Geometry: final body of the model. Coordinates: model frame, mm. Face numbers are marked on the shaded views. A direction names the side the tool comes from. Coordinates: 2 decimals unless noted, no trailing zeros. Loops run counter-clockwise (first coordinate to the right, second up) from the corner with the lowest first, then second, coordinate; pieces in that order, holes last. Notation, with made-up numbers: (3.25, 18) - (25.25, 18) arc R16 cw to (25.25, 23) - close; hole circle Ø3 at (23, 14.5). An arc over 180 degrees is marked (long way). Put each result on its own line as item: value. Start each with the question number.
1) Reachability of the marked faces 5, 6 and 7 from +Z, -Z, +X, -X, +Y, -Y: full face, straight path, thin tool, end or side. Return the list, or none.
2) Section C-C on y = 11. Output: boundary loops of the cut face in (x, z), and give its area (3 significant figures).
3) Material intervals for line 1 along Z through (x, y) = (-5.5, 9.25); line 2 along X through (y, z) = (18, 1), sorted ascending. Write a range as from..to.
4) Section D-D on z = 0. Output: boundary loops of the cut face in (x, y).
5) Section A-A on z = 14.5. Output: boundary loops of the cut face in (x, y).
6) Section B-B on x = -9.5. Output: boundary loops of the cut face in (y, z), and give its area (3 significant figures).
7) Draft query along Z for the marked faces 1, 2, 3 and 4. Return one class per face: +Z half, -Z half, draft (parallel to the pull), parting line (faces both ways), or undercut.
8) Contact query for flat-ended pins moving along their axis: pin 1 Ø23.5 at (x, z) = (-9, 0) entering from +Y; pin 2 Ø22 at (x, z) = (-0.5, 25.5) entering from +Y; pin 3 Ø3 at (x, y) = (-11.5, 21.5) entering from -Z. Output: stop coordinate, or through.
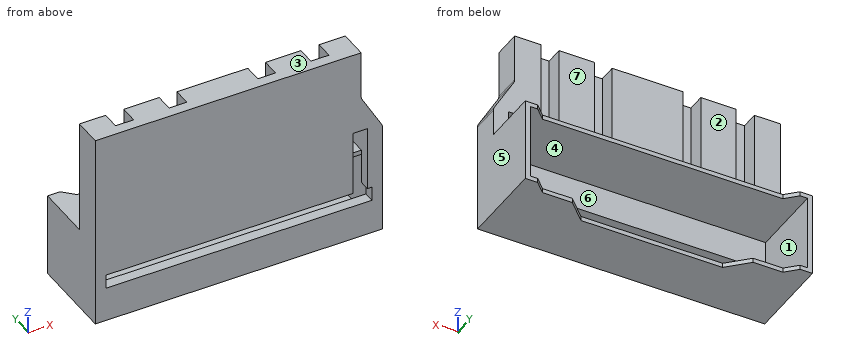
```python
from build123d import *

# Parameters (mm, degrees)
BOSS_EXTRUDE1_DEPTH = 3
SKETCH7_W           = 81
SKETCH7_H           = 23.7
SKETCH7_W_2         = 78.2
SKETCH7_H_2         = 21.2
BOSS_EXTRUDE4_DEPTH = 23.5
CUT_EXTRUDE7_START  = -22.45
CUT_EXTRUDE7_DEPTH  = 22.45
CUT_EXTRUDE8_DEPTH  = 4
CUT_EXTRUDE9_DEPTH  = 4
SKETCH17_W          = 7.4
SKETCH17_H          = 32.3
SKETCH17_W_2        = 10
SKETCH17_W_3        = 20
BOSS_EXTRUDE5_DEPTH = 5
CUT_EXTRUDE10_DEPTH = 1.25
FILLET1_R           = 2


with BuildPart() as part:
    # Sketch1 → Boss-Extrude1 (new body)
    with BuildSketch(Plane(origin=(0, 0, 0), x_dir=(1, 0, 0), z_dir=(0, 1, 0))):
        Polygon((-40.5, -11.85), (-40.5, 11.85), (0, 11.85), (40.5, 11.85), (40.5, -11.85), (40.5, -19.85), (34.5, -30.242304845), (34.5, -44.15), (-40.5, -44.15), align=None)
    extrude(amount=BOSS_EXTRUDE1_DEPTH)

    # Sketch7 → Boss-Extrude4 (add)
    with BuildSketch(Plane(origin=(0, 3, 0), x_dir=(1, 0, 0), z_dir=(0, 1, 0))):
        Rectangle(SKETCH7_W, SKETCH7_H)
        Rectangle(SKETCH7_W_2, SKETCH7_H_2, mode=Mode.SUBTRACT)
    extrude(amount=BOSS_EXTRUDE4_DEPTH)

    # Sketch16 → Cut-Extrude7 (cut)
    with BuildSketch(Plane(origin=(0, 0, -11.85), x_dir=(-1, 0, 0), z_dir=(0, 0, -1)).offset(CUT_EXTRUDE7_START)):
        Polygon((-40.5, 26.5), (40.5, 26.5), (40.5, 24.1), (37, 24.1), (33.9, 21), (25.5, 21), (20, 15.5), (-20, 15.5), (-25.5, 21), (-33.9, 21), (-37, 24.1), (-40.5, 24.1), align=None)
    extrude(amount=CUT_EXTRUDE7_DEPTH, mode=Mode.SUBTRACT)

    # Sketch8 → Cut-Extrude8 (cut)
    with BuildSketch(Plane(origin=(0, 3, 0), x_dir=(1, 0, 0), z_dir=(0, 1, 0))):
        Polygon((33.5, -2), (37.5, -2), (37.5, 2), (-37.5, 2), (-37.5, -2), align=None)
    extrude(amount=-CUT_EXTRUDE8_DEPTH, mode=Mode.SUBTRACT)

    # Sketch14 → Cut-Extrude9 (cut)
    with BuildSketch(Plane(origin=(0, 3, 0), x_dir=(1, 0, 0), z_dir=(0, 1, 0))):
        Polygon((36.25, -11.85), (36.25, -20.35), (32.25, -20.35), (32.25, -11.85), (32.25, 0.15), (36.25, 0.15), align=None)
    extrude(amount=-CUT_EXTRUDE9_DEPTH, mode=Mode.SUBTRACT)

    # Sketch17 → Boss-Extrude5 (add)
    with BuildSketch(Plane(origin=(0, 3, 0), x_dir=(1, 0, 0), z_dir=(0, 1, 0))):
        Polygon((32.25, -20.35), (36.25, -20.35), (36.25, -11.85), (40.5, -11.85), (40.5, -19.85), (34.5, -30.242304845), (34.5, -44.15), (27.1, -44.15), (27.1, -11.85), (32.25, -11.85), align=None)
        with Locations((-36.8, -28)):
            Rectangle(SKETCH17_W, SKETCH17_H)
        with Locations((-23, -28)):
            Rectangle(SKETCH17_W_2, SKETCH17_H)
        with Locations((-3, -28)):
            Rectangle(SKETCH17_W_3, SKETCH17_H)
        with Locations((17, -28)):
            Rectangle(SKETCH17_W_2, SKETCH17_H)
    extrude(amount=BOSS_EXTRUDE5_DEPTH)

    # Sketch18 → Cut-Extrude10 (cut)
    with BuildSketch(Plane(origin=(0, 0, 10.6), x_dir=(-1, 0, 0), z_dir=(0, 0, -1))):
        Polygon((40.5, 26.5), (40.5, 24.1), (37, 24.1), (33.9, 21), (-33.9, 21), (-37, 24.1), (-40.5, 24.1), (-40.5, 26.5), align=None)
    extrude(amount=-CUT_EXTRUDE10_DEPTH, mode=Mode.SUBTRACT)

    # Fillet1
    fillet1_edges = [part.edges().sort_by_distance(p)[0] for p in [
        (40.5, 4, 19.85),
        (34.5, 4, 30.242304845),
    ]]
    fillet(fillet1_edges, radius=FILLET1_R)


solid = part.part
```
Answer block:
1. face 5: +Z, -Z, +X, +Y, -Y
1. face 6: +Y
1. face 7: +Z, +X, -X, +Y
2. outline: (-40.5, -11.85) - (40.5, -11.85) - (40.5, 11.85) - (-40.5, 11.85) - close; hole (-39.1, -10.6) - (39.1, -10.6) - (39.1, 10.6) - (-39.1, 10.6) - close
2. area: 262 mm²
3. line 1: z = -11.85..-10.6, 10.6..11.85
3. line 2: x = -40.5..-39.1, 39.1..40.5
4. outline: (-40.5, 0) - (-37.5, 0) - (-37.5, 3) - (-39.1, 3) - (-39.1, 24.1) - (-40.5, 24.1) - close; (37.5, 0) - (40.5, 0) - (40.5, 24.1) - (39.1, 24.1) - (39.1, 3) - (37.5, 3) - close
5. outline: (-40.5, 0) - (32.25, 0) - (32.25, 8) - (27.1, 8) - (27.1, 3) - (22, 3) - (22, 8) - (12, 8) - (12, 3) - (7, 3) - (7, 8) - (-13, 8) - (-13, 3) - (-18, 3) - (-18, 8) - (-28, 8) - (-28, 3) - (-33.1, 3) - (-33.1, 8) - (-40.5, 8) - close; (36.25, 0) - (40.5, 0) - (40.5, 8) - (36.25, 8) - close
6. outline: (0, -11.85) - (15.5, -11.85) - (15.5, -10.6) - (3, -10.6) - (3, -2) - (0, -2) - close; (0, 2) - (3, 2) - (3, 10.6) - (21, 10.6) - (21, 11.85) - (8, 11.85) - (8, 44.15) - (0, 44.15) - close
6. area: 356 mm²
7. face 1: undercut
7. face 2: draft
7. face 3: +Z half
7. face 4: undercut
8. pin 1: stops at y = 21
8. pin 2: stops at y = 8
8. pin 3: stops at z = 10.6
